Here's how the part is built. I have some questions about the finished solid (model axes, mm). A direction names the side the tool comes from. Round coordinates to 2 decimals unless told otherwise and drop trailing zeros. Write each loop counter-clockwise with the first axis right and the second up, starting at its lowest first coordinate (ties: lowest second). Pieces come first, ordered by that corner, then holes. Notation, with made-up numbers: (-13.5, -31.75) - (12.5, -31.75) arc R18 cw to (12.5, -27.75) - close; hole circle Ø7 at (73, 46). An arc over 180 degrees is marked (long way). Write item = value, one per line. Start each with the question number.
Item 1: If we section it at B-B (z = 5.25): Give the number of separate pieces and of enclosed holes in the cut face, and give its area (3 significant figures).
Item 2: If we section it at D-D (y = 16.5): Please give me the cut outline in (x, z) (3 decimals).
Item 3: For P1, Ø1.5, axis at x = -33, y = 15.5, coming from the +Z side; P2, Ø8, axis at x = 38.1, y = 7.14, coming from the +Z side; P3, Ø3.5, axis at x = -28.58, y = 4.76, coming from the -Z side, each with a flat end and sliding along its axis, tell me the tip position at first contact or that it passes through.
Item 4: If I drill on line 1 along Y through (x, z) = (-1, 2.75); line 2 along X through (y, z) = (3, 3.5); line 3 along X through (y, z) = (2.75, 2.5), over which ranges is the centre line in solid material (lowest first)? Write a range as [from, to].
Item 5: Thinking about a two-plate mould opening in X: for faces 1 (the face through (-39.456, 15.224, 3.219)), 2 (the face through (-1, 12, 6.35)), 3 (the face through (26.99, 4.83, 3.13)), 4 (the face through (-37, 11, 2.381)), which applies, pulls with the +X half, pulls with the -X half, needs draft (parallel to the pull), parting line crosses it, or undercut?
Item 6: If we section it at A-A (x = 19.05): Please give me the cut outline in (y, z), and give its area (3 significant figures).
Item 7: If we section it at C-C (x = -8): Please give me the cut outline in (y, z), and give its area (3 significant figures).
Item 8: Which directions (+Z, -Z, +X, -X, +Y, -Y) give clear straight access to the entire face, cutting with the end or side of a thin tool? Please do faces 5 (the face through (-44.45, 6, 3)), 6 (the face through (39, 11, 2.381)), 7 (the face through (-0.15, 11.31, 3.22)), 8 (the face through (-28.575, 13, 3)).
```python
from build123d import *

# Parameters (mm, degrees)
SKETCH1_W          = 88.9
SKETCH1_H          = 19.05
BASE_EXTRUDE_DEPTH = 6.35
CUT_EXTRUDE1_DEPTH = 49.775275499
CUT_EXTRUDE3_DEPTH = 49.775275499
CUT_EXTRUDE4_DEPTH = 49.775275499
CUT_EXTRUDE5_DEPTH = 49.775275499
FILLET1_R          = 3.175
HOLE1_D            = 7.14375
HOLE1_CBORE_D      = 10.31875
HOLE1_CBORE_DEPTH  = 3.96875
LPATTERN1_COUNT    = 2
LPATTERN1_PITCH    = 76.2
HOLE2_OUTLINE_R    = 1.5875
HOLE2_DEPTH        = 6.35
HOLE3_OUTLINE_R    = 1.5875
HOLE3_DEPTH        = 6.35
LPATTERN2_COUNT    = 2
LPATTERN2_PITCH    = 57.15


# Read off the part's stored shape, not the designer's step: Hole2, Hole3
with BuildPart() as part:
    # Sketch1 → Base-Extrude (new body)
    with BuildSketch(Plane.XY):
        with Locations((0, 9.525)):
            Rectangle(SKETCH1_W, SKETCH1_H)
    extrude(amount=BASE_EXTRUDE_DEPTH)

    # Sketch2 → Cut-Extrude1 (cut, through all)
    with BuildSketch(Plane.XY.offset(6.35)):
        Polygon((44.45, 14.2875), (25.4, 19.05), (44.45, 19.05), align=None)
    extrude(amount=-CUT_EXTRUDE1_DEPTH, mode=Mode.SUBTRACT)

    # Sketch4 → Cut-Extrude3 (cut, through all)
    with BuildSketch(Plane.XY.offset(6.35)):
        Polygon((-231.275885049, -20.742353447), (-44.45, 14.2875), (-19.05, 19.05), (167.775885049, 54.079853447), (97.716178156, 427.731623544), (-301.335591942, 352.909416651), align=None)
    extrude(amount=-CUT_EXTRUDE3_DEPTH, mode=Mode.SUBTRACT)

    # Sketch5 → Cut-Extrude4 (cut, through all)
    with BuildSketch(Plane.XY.offset(6.35)):
        Polygon((-36.984386732, 15.687302488), (-28.575, 8.262261056), (-28.575, 17.2640625), align=None)
    extrude(amount=-CUT_EXTRUDE4_DEPTH, mode=Mode.SUBTRACT)

    # Sketch6 → Cut-Extrude5 (cut, through all)
    with BuildSketch(Plane.XY.offset(6.35)):
        with BuildLine():
            ThreePointArc((-10.884660771, 12.84067681), (0, 11.3109375), (10.884660771, 12.84067681))
            ThreePointArc((10.884660771, 12.84067681), (15.057262416, 10.52776595), (12.744351556, 6.355164305))
            ThreePointArc((12.744351556, 6.355164305), (0, 4.5640625), (-12.744351556, 6.355164305))
            ThreePointArc((-12.744351556, 6.355164305), (-15.057262416, 10.52776595), (-10.884660771, 12.84067681))
        make_face()
    extrude(amount=-CUT_EXTRUDE5_DEPTH, mode=Mode.SUBTRACT)

    # Fillet1
    fillet1_edges = [part.edges().sort_by_distance(p)[0] for p in [
        (44.45, 14.2875, 3.175),
        (25.4, 19.05, 3.175),
        (-19.05, 19.05, 3.175),
        (-44.45, 14.2875, 3.175),
    ]]
    fillet(fillet1_edges, radius=FILLET1_R)

    # Hole1 (through all)
    with Locations(Plane.XY.offset(6.35)):
        with Locations((38.1, 7.14375)):
            hole1 = CounterBoreHole(HOLE1_D / 2, HOLE1_CBORE_D / 2, HOLE1_CBORE_DEPTH)

    # LPattern1: Hole1 ×2
    with Locations(*[(-i * LPATTERN1_PITCH, 0, 0) for i in range(1, LPATTERN1_COUNT)]):
        add(hole1, mode=Mode.SUBTRACT)

    # Hole2 outline → Hole2 (cut)
    with BuildSketch(Plane.XY):
        with Locations((28.575, 4.7625)):
            Circle(HOLE2_OUTLINE_R)
    hole2 = extrude(amount=HOLE2_DEPTH, mode=Mode.SUBTRACT)

    # Hole3 outline → Hole3 (cut)
    with BuildSketch(Plane.XY):
        with Locations((19.05, 3.175)):
            Circle(HOLE3_OUTLINE_R)
    extrude(amount=HOLE3_DEPTH, mode=Mode.SUBTRACT)

    # LPattern2: Hole2 ×2
    with Locations(*[(-i * LPATTERN2_PITCH, 0, 0) for i in range(1, LPATTERN2_COUNT)]):
        add(hole2, mode=Mode.SUBTRACT)


solid = part.part
```
Reply:
q1.separate_pieces = 1
q1.enclosed_holes = 6
q1.area = 1,160 mm2
q2.outline = (-28.575, 0) - (35.6, 0) - (35.6, 6.35) - (-28.575, 6.35) - close
q3.P1 = through
q3.P2 = 2.38
q3.P3 = 0
q4.line_1 = [0, 4.57], [11.32, 19.05]
q4.line_2 = [-44.45, -41.17], [-35.03, 17.47], [20.63, 35.03], [41.17, 44.45]
q4.line_3 = [-44.45, -40.8], [-35.4, 17.52], [20.58, 35.4], [40.8, 44.45]
q5.face_1 = pulls with the -X half
q5.face_2 = needs draft
q5.face_3 = undercut
q5.face_4 = undercut
q6.outline = (0, 0) - (1.59, 0) - (1.59, 6.35) - (0, 6.35) - close; (4.76, 0) - (19.05, 0) - (19.05, 6.35) - (4.76, 6.35) - close
q6.area = 101 mm2
q7.outline = (0, 0) - (5.26, 0) - (5.26, 6.35) - (0, 6.35) - close; (12.13, 0) - (19.05, 0) - (19.05, 6.35) - (12.13, 6.35) - close
q7.area = 77.4 mm2
q8.face_5 = +Z, -Z, -X, +Y, -Y
q8.face_6 = +Z
q8.face_7 = +Z, -Z
q8.face_8 = +Z, -Z, +Y
